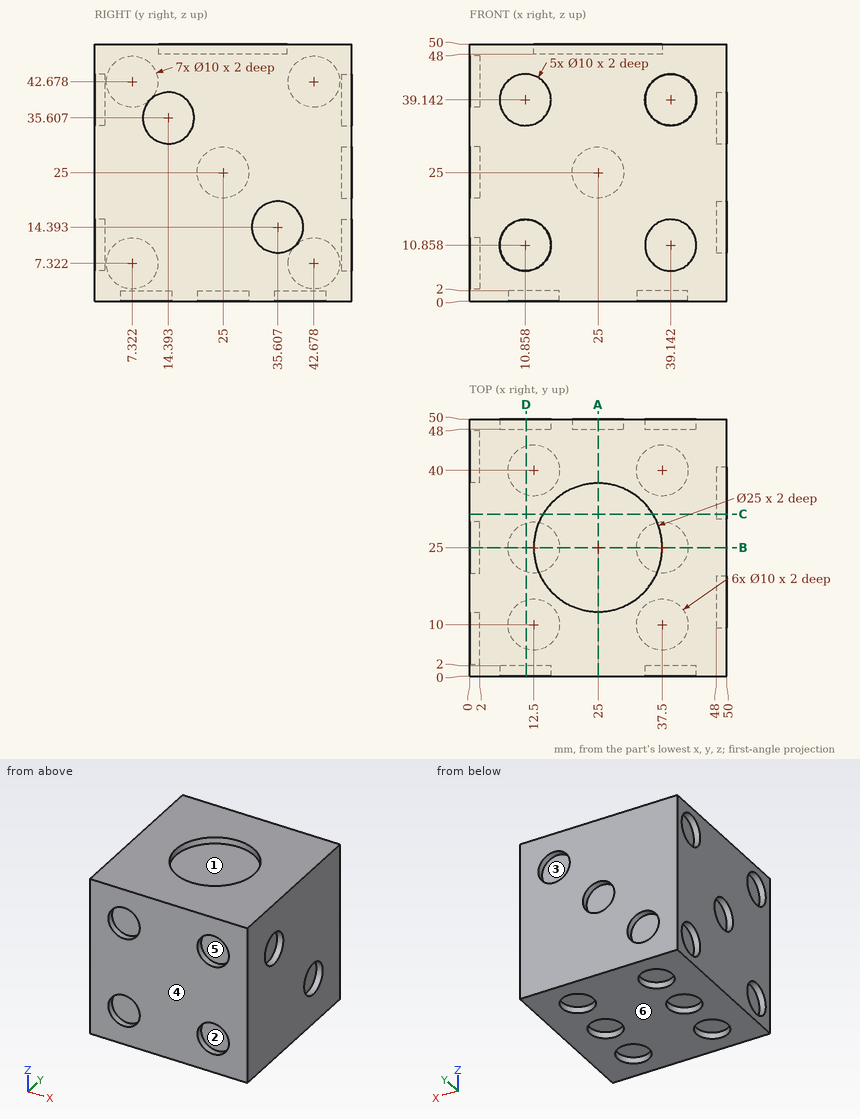
Print and shaded views of the part. All mm, measured from the part's lowest x, y and z. A direction names the side the tool comes from. Coordinates: 2 decimals unless noted, no trailing zeros. Order: outer loops, then holes, each group sorted by start corner. A loop starts at its lowest first (then second) coordinate and runs counter-clockwise, first axis right, second up.
Item 1: Saw through at B-B on y = 25. List the corners of the cut face in (x, z).
Filled in:
outline: (0, 0) - (7.5, 0) - (7.5, 2) - (17.5, 2) - (17.5, 0) - (32.5, 0) - (32.5, 2) - (42.5, 2) - (42.5, 0) - (50, 0) - (50, 50) - (37.5, 50) - (37.5, 48) - (12.5, 48) - (12.5, 50) - (0, 50) - (0, 30) - (2, 30) - (2, 20) - (0, 20) - close
Item 2: Drill centre lines: L1, parallel to Y at x = 25, z = 48.9; L2, parallel to Y at x = 35.5, z = 11.5; L3, parallel to Z at x = 22, y = 21. Where is each one in solid material? Low to high.
Filled in:
L1: y = 0 to 12.5, 37.5 to 50
L2: y = 2 to 50
L3: z = 0 to 48
Item 3: Saw through at A-A on x = 25. List the corners of the cut face in (y, z).
Filled in:
outline: (0, 0) - (50, 0) - (50, 20) - (48, 20) - (48, 30) - (50, 30) - (50, 50) - (37.5, 50) - (37.5, 48) - (12.5, 48) - (12.5, 50) - (0, 50) - close
Item 4: Drop flat-ended pins along their axis: pin 1 Ø3 at (x, z) = (26.5, 26) entering from +Y; pin 2 Ø3 at (y, z) = (25.5, 24) entering from -X; pin 3 Ø6 at (x, y) = (12.5, 40) entering from -Z. Give the stop position or say it passes through.
Filled in:
pin 1: stops at y = 48
pin 2: stops at x = 2
pin 3: stops at z = 2
Item 5: Saw through at D-D on x = 11. List the corners of the cut face in (y, z), then the cut area to 3 significant figures.
Filled in:
outline: (0, 0) - (5.23, 0) - (5.23, 2) - (14.77, 2) - (14.77, 0) - (20.23, 0) - (20.23, 2) - (29.77, 2) - (29.77, 0) - (35.23, 0) - (35.23, 2) - (44.77, 2) - (44.77, 0) - (50, 0) - (50, 5.86) - (48, 5.86) - (48, 15.86) - (50, 15.86) - (50, 50) - (0, 50) - (0, 44.14) - (2, 44.14) - (2, 34.14) - (0, 34.14) - (0, 15.86) - (2, 15.86) - (2, 5.86) - (0, 5.86) - close
area: 2,380 mm2
Item 6: Tool access for the marked faces 1, 2 and 3: list every direction of +Z, -Z, +X, -X, +Y, -Y with a clear straight run to the whole face (end or side of a thin tool).
Filled in:
face 1: +Z
face 2: -Y
face 3: +Y
Item 7: Mould opens along Z. For the marked faces 4, 5 and 6 say: released by +Z, released by -Z, zero draft, split by the parting line, or undercut.
Filled in:
face 4: zero draft
face 5: undercut
face 6: released by -Z
Item 8: Saw through at C-C on y = 31.5. List the corners of the cut face in (x, z) (1 decimal), then the cut area to 3 significant figures.
Filled in:
outline: (0, 0) - (50, 0) - (50, 11.5) - (48, 11.5) - (48, 17.2) - (50, 17.2) - (50, 50) - (35.7, 50) - (35.7, 48) - (14.3, 48) - (14.3, 50) - (0, 50) - close
area: 2,450 mm2
